Could you check a few things on this model? Use its own coordinates, in mm. A direction names the side the tool comes from. Round coordinates to 2 decimals unless told otherwise and drop trailing zeros. Loops run counter-clockwise (first coordinate to the right, second up) from the corner with the lowest first, then second, coordinate; pieces in that order, holes last. Notation, with made-up numbers: (64.25, 26) -> (105.25, 26) arc R28 ccw to (105.25, 50) -> close; hole circle Ø4 at (-36.75, 41.5). An arc over 180 degrees is marked (long way). Put each result on its own line as item: value. Start each with the question number.
1. If we mould it in two halves opening along Z, with no side actions, what happens to faces 3 (the cylindrical face through (347.57, 1.5, -51.44)), 4 (the flat face through (692.15, 3, -46)), 5 (the flat face through (50, 12, -81.407))? For each: pulls with the +Z half, pulls with the -Z half, needs draft (parallel to the pull), parting line crosses it, or undercut.
2. Which directions (+Z, -Z, +X, -X, +Y, -Y) give clear straight access to the entire face, cutting with the end or side of a thin tool? Please do faces 1 (the flat face through (351, 19, 0)), 2 (the flat face through (644, 12, -81.407)).
3. Imagine slicing it at C-C, the plane x = 370.5. Please give me the cut outline in (y, z) (3 decimals).
4. I need wall thicknesses on line 1 (Z direction, x = 81, y = 15) (3 decimals); line 2 (Z direction, x = 495, y = 3); line 3 (Z direction, x = 450.5, y = 30.5) (3 decimals). Which ranges of each line are inside material? Lowest first, please. Write a range as [from, to].
5. Imagine slicing it at B-B, the plane x = 465.5. Please give me the cut outline in (y, z) (3 decimals).
6. Imagine slicing it at A-A, the plane z = -60. Please give me the cut outline in (x, y) (3 decimals).
7. I'm going to push flat-ended pins straight in: P1, Ø4, axis at x = 545, y = 38, coming from the +Z side; P2, Ø1.6, axis at x = 653.5, z = -83.5, coming from the +Y side; P3, Ø4, axis at x = 215.9, z = -5.842, coming from the +Y side. Where does each tip first touch, or does it pass through?
```python
from build123d import *

# Parameters (mm, degrees)
SKETCH1_W                    = 692.15
SKETCH1_H                    = 84.582
BOSS_EXTRUDE1_DEPTH          = 53.975
SKETCH2_W                    = 84.582
SKETCH2_H                    = 50.8
CUT_EXTRUDE1_DEPTH           = 700.38475666
SKETCH3_W                    = 692.15
SKETCH3_H                    = 3.175
BOSS_EXTRUDE2_DEPTH          = 31.75
M2_CLEARANCE_HOLE1_D         = 2.54
M5_START                     = -84.582
M5_CLEARANCE_HOLE2_OUTLINE_R = 2.667
M5_CLEARANCE_HOLE2_DEPTH     = 84.582
CHAMFER1_SIZE                = 3.175
FILLET1_R                    = 0.762
FILLET2_R                    = 3.937
CUT_EXTRUDE7_DEPTH           = 58.674
CUT_EXTRUDE7_DEPTH_BACK      = 182.626
CUT_EXTRUDE8_DEPTH           = 66.802
CUT_EXTRUDE8_DEPTH_BACK      = 191.516
CUT_EXTRUDE9_REACH           = 701.385
CUT_EXTRUDE10_DEPTH          = 700.38475666
F_10_32_TAPPED_HOLE1_D       = 4.0386
F_10_32_TAPPED_HOLE1_DEPTH   = 13.716
F_10_32_TAPPED_HOLE1_TIP     = 1.213317848
SKETCH22_R                   = 5.159375
CUT_EXTRUDE11_DEPTH          = 3.175


# Read off the part's stored shape, not the designer's step: M5 Clearance Hole2
with BuildPart() as part:
    # Sketch1 → Boss-Extrude1 (new body)
    with BuildSketch(Plane(origin=(0, 53.975, 0), x_dir=(1, 0, 0), z_dir=(0, 1, 0))):
        with Locations((346.075, 42.291)):
            Rectangle(SKETCH1_W, SKETCH1_H)
    extrude(amount=-BOSS_EXTRUDE1_DEPTH)

    # Sketch2 → Cut-Extrude1 (cut, through all)
    with BuildSketch(Plane(origin=(692.15, 0, 0), x_dir=(0, 0, -1), z_dir=(1, 0, 0))):
        with Locations((39.116, 28.575)):
            Rectangle(SKETCH2_W, SKETCH2_H)
    extrude(amount=-CUT_EXTRUDE1_DEPTH, mode=Mode.SUBTRACT)

    # Sketch3 → Boss-Extrude2 (add)
    with BuildSketch(Plane(origin=(0, 3.175, 0), x_dir=(-1, 0, 0), z_dir=(0, 1, 0))):
        with Locations((-346.075, -1.5875)):
            Rectangle(SKETCH3_W, SKETCH3_H)
    extrude(amount=BOSS_EXTRUDE2_DEPTH)

    # M2 Clearance Hole1 (through all)
    with Locations(Plane(origin=(0, 3.175, 0), x_dir=(1, 0, 0), z_dir=(0, 1, 0))):
        with Locations((215.9, 5.842), (215.9, 72.39)):
            Hole(M2_CLEARANCE_HOLE1_D / 2)

    # M5 Clearance Hole2 outline → M5 Clearance Hole2 (cut)
    with BuildSketch(Plane.XY.offset(M5_START)):
        with Locations((683.006, 42.037)):
            Circle(M5_CLEARANCE_HOLE2_OUTLINE_R)
        with Locations((670.306, 42.037)):
            Circle(M5_CLEARANCE_HOLE2_OUTLINE_R)
        with Locations((657.606, 42.037)):
            Circle(M5_CLEARANCE_HOLE2_OUTLINE_R)
        with Locations((644.906, 42.037)):
            Circle(M5_CLEARANCE_HOLE2_OUTLINE_R)
        with Locations((632.206, 42.037)):
            Circle(M5_CLEARANCE_HOLE2_OUTLINE_R)
        with Locations((619.506, 42.037)):
            Circle(M5_CLEARANCE_HOLE2_OUTLINE_R)
        with Locations((594.106, 42.037)):
            Circle(M5_CLEARANCE_HOLE2_OUTLINE_R)
        with Locations((581.406, 42.037)):
            Circle(M5_CLEARANCE_HOLE2_OUTLINE_R)
        with Locations((568.706, 42.037)):
            Circle(M5_CLEARANCE_HOLE2_OUTLINE_R)
        with Locations((556.006, 42.037)):
            Circle(M5_CLEARANCE_HOLE2_OUTLINE_R)
        with Locations((543.306, 42.037)):
            Circle(M5_CLEARANCE_HOLE2_OUTLINE_R)
        with Locations((530.606, 42.037)):
            Circle(M5_CLEARANCE_HOLE2_OUTLINE_R)
        with Locations((517.906, 42.037)):
            Circle(M5_CLEARANCE_HOLE2_OUTLINE_R)
        with Locations((505.206, 42.037)):
            Circle(M5_CLEARANCE_HOLE2_OUTLINE_R)
        with Locations((492.506, 42.037)):
            Circle(M5_CLEARANCE_HOLE2_OUTLINE_R)
        with Locations((479.806, 42.037)):
            Circle(M5_CLEARANCE_HOLE2_OUTLINE_R)
        with Locations((467.106, 42.037)):
            Circle(M5_CLEARANCE_HOLE2_OUTLINE_R)
        with Locations((454.406, 42.037)):
            Circle(M5_CLEARANCE_HOLE2_OUTLINE_R)
        with Locations((441.706, 42.037)):
            Circle(M5_CLEARANCE_HOLE2_OUTLINE_R)
        with Locations((429.006, 42.037)):
            Circle(M5_CLEARANCE_HOLE2_OUTLINE_R)
        with Locations((416.306, 42.037)):
            Circle(M5_CLEARANCE_HOLE2_OUTLINE_R)
        with Locations((403.606, 42.037)):
            Circle(M5_CLEARANCE_HOLE2_OUTLINE_R)
        with Locations((390.906, 42.037)):
            Circle(M5_CLEARANCE_HOLE2_OUTLINE_R)
        with Locations((378.206, 42.037)):
            Circle(M5_CLEARANCE_HOLE2_OUTLINE_R)
        with Locations((365.506, 42.037)):
            Circle(M5_CLEARANCE_HOLE2_OUTLINE_R)
        with Locations((352.806, 42.037)):
            Circle(M5_CLEARANCE_HOLE2_OUTLINE_R)
        with Locations((340.106, 42.037)):
            Circle(M5_CLEARANCE_HOLE2_OUTLINE_R)
        with Locations((327.406, 42.037)):
            Circle(M5_CLEARANCE_HOLE2_OUTLINE_R)
        with Locations((314.706, 42.037)):
            Circle(M5_CLEARANCE_HOLE2_OUTLINE_R)
        with Locations((302.006, 42.037)):
            Circle(M5_CLEARANCE_HOLE2_OUTLINE_R)
        with Locations((289.306, 42.037)):
            Circle(M5_CLEARANCE_HOLE2_OUTLINE_R)
        with Locations((276.606, 42.037)):
            Circle(M5_CLEARANCE_HOLE2_OUTLINE_R)
        with Locations((263.906, 42.037)):
            Circle(M5_CLEARANCE_HOLE2_OUTLINE_R)
        with Locations((251.206, 42.037)):
            Circle(M5_CLEARANCE_HOLE2_OUTLINE_R)
        with Locations((238.506, 42.037)):
            Circle(M5_CLEARANCE_HOLE2_OUTLINE_R)
        with Locations((225.806, 42.037)):
            Circle(M5_CLEARANCE_HOLE2_OUTLINE_R)
        with Locations((213.106, 42.037)):
            Circle(M5_CLEARANCE_HOLE2_OUTLINE_R)
        with Locations((200.406, 42.037)):
            Circle(M5_CLEARANCE_HOLE2_OUTLINE_R)
        with Locations((187.706, 42.037)):
            Circle(M5_CLEARANCE_HOLE2_OUTLINE_R)
        with Locations((175.006, 42.037)):
            Circle(M5_CLEARANCE_HOLE2_OUTLINE_R)
        with Locations((162.306, 42.037)):
            Circle(M5_CLEARANCE_HOLE2_OUTLINE_R)
        with Locations((149.606, 42.037)):
            Circle(M5_CLEARANCE_HOLE2_OUTLINE_R)
        with Locations((136.906, 42.037)):
            Circle(M5_CLEARANCE_HOLE2_OUTLINE_R)
        with Locations((124.206, 42.037)):
            Circle(M5_CLEARANCE_HOLE2_OUTLINE_R)
        with Locations((683.006, 16.637)):
            Circle(M5_CLEARANCE_HOLE2_OUTLINE_R)
        with Locations((619.506, 16.637)):
            Circle(M5_CLEARANCE_HOLE2_OUTLINE_R)
        with Locations((606.806, 16.637)):
            Circle(M5_CLEARANCE_HOLE2_OUTLINE_R)
        with Locations((594.106, 16.637)):
            Circle(M5_CLEARANCE_HOLE2_OUTLINE_R)
        with Locations((111.506, 42.037)):
            Circle(M5_CLEARANCE_HOLE2_OUTLINE_R)
        with Locations((98.806, 42.037)):
            Circle(M5_CLEARANCE_HOLE2_OUTLINE_R)
        with Locations((73.406, 42.037)):
            Circle(M5_CLEARANCE_HOLE2_OUTLINE_R)
        with Locations((60.706, 42.037)):
            Circle(M5_CLEARANCE_HOLE2_OUTLINE_R)
        with Locations((48.006, 42.037)):
            Circle(M5_CLEARANCE_HOLE2_OUTLINE_R)
        with Locations((35.306, 42.037)):
            Circle(M5_CLEARANCE_HOLE2_OUTLINE_R)
        with Locations((22.606, 42.037)):
            Circle(M5_CLEARANCE_HOLE2_OUTLINE_R)
        with Locations((9.906, 42.037)):
            Circle(M5_CLEARANCE_HOLE2_OUTLINE_R)
        with Locations((98.806, 16.637)):
            Circle(M5_CLEARANCE_HOLE2_OUTLINE_R)
        with Locations((86.106, 16.637)):
            Circle(M5_CLEARANCE_HOLE2_OUTLINE_R)
        with Locations((73.406, 16.637)):
            Circle(M5_CLEARANCE_HOLE2_OUTLINE_R)
        with Locations((9.906, 16.637)):
            Circle(M5_CLEARANCE_HOLE2_OUTLINE_R)
    extrude(amount=M5_CLEARANCE_HOLE2_DEPTH, mode=Mode.SUBTRACT)

    # Chamfer1
    chamfer1_edges = [part.edges().sort_by_distance(p)[0] for p in [
        (692.15, 53.975, -82.9945),
        (0, 34.925, -1.5875),
        (692.15, 34.925, -1.5875),
        (0, 53.975, -82.9945),
    ]]
    chamfer(chamfer1_edges, length=CHAMFER1_SIZE)

    # Fillet1
    fillet1_edges = [part.edges().sort_by_distance(p)[0] for p in [
        (346.075, 3.175, -81.407),
        (346.075, 3.175, -3.175),
    ]]
    fillet(fillet1_edges, radius=FILLET1_R)

    # Fillet2
    fillet2_edges = [part.edges().sort_by_distance(p)[0] for p in [
        (346.075, 0, 0),
        (346.075, 0, -84.582),
    ]]
    fillet(fillet2_edges, radius=FILLET2_R)

    # Sketch15 → Cut-Extrude7 (cut, two sides: drawn at the far end of the back side and taken through both)
    with BuildSketch(Plane(origin=(0, 0, -84.582), x_dir=(-1, 0, 0), z_dir=(0, 0, -1)).offset(-CUT_EXTRUDE7_DEPTH_BACK)):
        with BuildLine():
            Line((-16.256, 27.686), (-16.256, 53.975))
            Line((-16.256, 53.975), (-67.056, 53.975))
            Line((-67.056, 53.975), (-67.056, 26.797))
            ThreePointArc((-67.056, 26.797), (-64.080204897, 19.612795103), (-56.896, 16.637))
            Line((-56.896, 16.637), (-26.416, 16.637))
            ThreePointArc((-26.416, 16.637), (-19.231795103, 19.612795103), (-16.256, 26.797))
            Line((-16.256, 26.797), (-16.256, 27.686))
        make_face()
    extrude(amount=CUT_EXTRUDE7_DEPTH + CUT_EXTRUDE7_DEPTH_BACK, mode=Mode.SUBTRACT)

    # Sketch16 → Cut-Extrude8 (cut, two sides: drawn at the far end of the back side and taken through both)
    with BuildSketch(Plane(origin=(0, 0, -84.582), x_dir=(-1, 0, 0), z_dir=(0, 0, -1)).offset(-CUT_EXTRUDE8_DEPTH_BACK)):
        with BuildLine():
            Line((-676.656, 27.3685), (-676.656, 26.797))
            ThreePointArc((-676.656, 26.797), (-673.680204897, 19.612795103), (-666.496, 16.637))
            Line((-666.496, 16.637), (-636.016, 16.637))
            ThreePointArc((-636.016, 16.637), (-628.831795103, 19.612795103), (-625.856, 26.797))
            Line((-625.856, 26.797), (-625.856, 53.975))
            Line((-625.856, 53.975), (-676.656, 53.975))
            Line((-676.656, 53.975), (-676.656, 27.3685))
        make_face()
    extrude(amount=CUT_EXTRUDE8_DEPTH + CUT_EXTRUDE8_DEPTH_BACK, mode=Mode.SUBTRACT)

    # Cut-Extrude9: up to this face of the body (flat: up to its plane)
    cut_extrude9_end = Plane(part.part.faces().sort_by_distance((346.012685058, 27.7502179, -81.407))[0])
    # Sketch17 → Cut-Extrude9 (cut, up to the picked face)
    with BuildSketch(Plane(origin=(0, 0, -84.582), x_dir=(-1, 0, 0), z_dir=(0, 0, -1)), mode=Mode.PRIVATE) as cut_extrude9_sk1:
        with BuildLine():
            Line((-600.456, 53.975), (-600.456, 10.287))
            ThreePointArc((-600.456, 10.287), (-598.596128061, 5.796871939), (-594.106, 3.937))
            Line((-594.106, 3.937), (-98.806, 3.937))
            ThreePointArc((-98.806, 3.937), (-94.315871939, 5.796871939), (-92.456, 10.287))
            Line((-92.456, 10.287), (-92.456, 53.975))
            Line((-92.456, 53.975), (-600.456, 53.975))
        make_face()
    cut_extrude9_tool1 = split(extrude(cut_extrude9_sk1.sketch, amount=-CUT_EXTRUDE9_REACH, mode=Mode.PRIVATE), bisect_by=cut_extrude9_end, keep=Keep.BOTH, mode=Mode.PRIVATE)
    add(cut_extrude9_tool1.solids().sort_by(Axis((346.456, 28.972079, -84.582), (0, 0, 1)))[0], mode=Mode.SUBTRACT)

    # Sketch18 → Cut-Extrude10 (cut, through all)
    with BuildSketch(Plane.XZ):
        with BuildLine():
            Line((246.845892421, -84.582), (445.304107579, -84.582))
            ThreePointArc((445.304107579, -84.582), (346.075, -51.435), (246.845892421, -84.582))
        make_face()
    extrude(amount=-CUT_EXTRUDE10_DEPTH, mode=Mode.SUBTRACT)

    # #10-32 Tapped Hole1
    with Locations(Plane(origin=(0, 0, 0), x_dir=(-1, 0, 0), z_dir=(0, -1, 0))):
        with Locations((-414.274, 32.893), (-414.274, 15.875), (-345.694, 15.841335103), (-345.694, 32.922547423), (-277.114, 32.952094846), (-277.114, 15.807670207)):
            Hole(F_10_32_TAPPED_HOLE1_D / 2, depth=F_10_32_TAPPED_HOLE1_DEPTH)
            with Locations((0, 0, -(F_10_32_TAPPED_HOLE1_DEPTH + F_10_32_TAPPED_HOLE1_TIP / 2))):  # 118° drill point
                Cone(0, F_10_32_TAPPED_HOLE1_D / 2, F_10_32_TAPPED_HOLE1_TIP, mode=Mode.SUBTRACT)

    # Sketch22 → Cut-Extrude11 (cut)
    with BuildSketch(Plane.XZ):
        with Locations(Location((161.98455352, -18.6699144, 0), (0, 0, 270))):
            Circle(SKETCH22_R)
        with Locations(Location((530.16544648, -18.6699144, 0), (0, 0, 270))):
            Circle(SKETCH22_R)
    extrude(amount=-CUT_EXTRUDE11_DEPTH, mode=Mode.SUBTRACT)


solid = part.part
```
Entries:
1. face 3: pulls with the -Z half
1. face 4: needs draft
1. face 5: undercut
2. face 1: +Z, +X, -X, +Y, -Y
2. face 2: +X, -X, +Y
3. outline: (0, -53.252) -> (3.175, -53.252) -> (3.175, -3.937) arc R0.762 cw to (3.937, -3.175) -> (34.925, -3.175) -> (34.925, 0) -> (3.937, 0) arc R3.937 ccw to (0, -3.937) -> close
4. line 1: [-84.582, -81.407], [-3.175, 0]
4. line 2: [-84.47, -0.11]
4. line 3: [-3.175, 0]
5. outline: (0, -80.645) arc R3.937 ccw to (3.937, -84.582) -> (3.937, -81.407) arc R0.762 cw to (3.175, -80.645) -> (3.175, -3.937) arc R0.762 cw to (3.937, -3.175) -> (34.925, -3.175) -> (34.925, 0) -> (3.937, 0) arc R3.937 ccw to (0, -3.937) -> close
6. outline: (0, 0) -> (293.589, 0) -> (293.589, 3.175) -> (0, 3.175) -> close; (398.561, 0) -> (692.15, 0) -> (692.15, 3.175) -> (398.561, 3.175) -> close
7. P1: through
7. P2: y = 16.64
7. P3: y = 3.18
